Design review of the part built by this model. Coordinates are the model's own, in mm. Round coordinates to 2 decimals unless told otherwise and drop trailing zeros. Order: outer loops, then holes, each group sorted by start corner. A loop starts at its lowest first (then second) coordinate and runs counter-clockwise, first axis right, second up. Notation, with made-up numbers: M 47,-0.5 L 54,-0.5 A19 cw 54,17.5 Z; hole C -13,54.25 d7. An arc over 180 degrees is marked long. Write each question's results on one line, items separated by ' | '. Start each with the question number.
Item 1: Clearance check with a flat-ended pin moving along its axis: pin 1 (3.5 mm diameter, centred on x = -29.5, z = 36.51, fed in from -Y). State where the tip first meets the part, or that it passes through.
Item 2: Take a section at B-B, the plane z = 38.1. Write out the cut boundary in (x, y).
Item 3: Take a section at D-D, the plane y = 2.5. Count the separate pieces of the cut face and the enclosed holes in it, plus the area to 3 significant figures.
Item 4: Take a section at A-A, the plane x = 50.8. Write out the cut boundary in (y, z).
Item 5: Wall thickness on line 1 (Z direction, x = -34.5, y = 3.75); line 2 (Z direction, x = -29.5, y = 2.25); line 3 (X direction, y = 4.5, z = -3): over which ranges is each line inside the solid? List them lowest first. Write a range as [from, to].
Item 6: Take a section at C-C, the plane x = -29.5. Write out the cut boundary in (y, z).
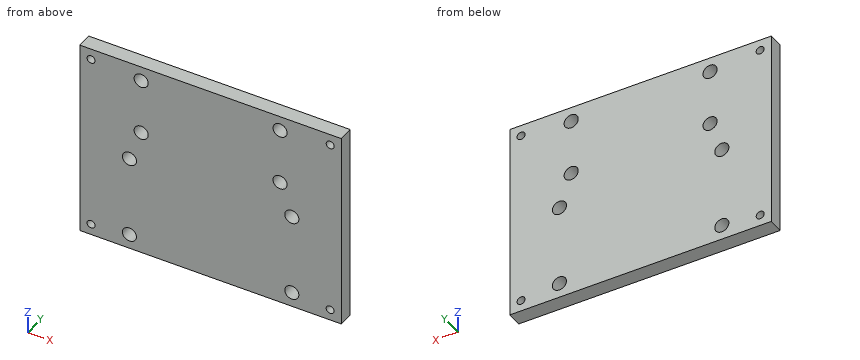
```python
from build123d import *

# Parameters (mm, degrees)
SKETCH1_W            = 111.125
SKETCH1_H            = 85.725
BOSS_EXTRUDE1_DEPTH  = 6.35
M3_CLEARANCE_HOLE1_D = 3.4
SKETCH3_R            = 3
CUT_EXTRUDE1_DEPTH   = 7.35


with BuildPart() as part:
    # Sketch1 → Boss-Extrude1 (new body)
    with BuildSketch(Plane(origin=(0, 0, 0), x_dir=(1, 0, 0), z_dir=(0, 1, 0))):
        Rectangle(SKETCH1_W, SKETCH1_H)
    extrude(amount=BOSS_EXTRUDE1_DEPTH)

    # M3 Clearance Hole1 (through all)
    with Locations(Plane(origin=(-50.8, 0, 38.1), x_dir=(0, 0, -1), z_dir=(0, -1, 0))):
        with Locations((0, 0), (0, 101.6), (76.2, 0), (76.2, 101.6)):
            Hole(M3_CLEARANCE_HOLE1_D / 2)

    # Sketch3 → Cut-Extrude1 (cut, through all)
    with BuildSketch(Plane(origin=(0, 6.35, 0), x_dir=(1, 0, 0), z_dir=(0, 1, 0))):
        with Locations((-34.5, 36.5125)):
            Circle(SKETCH3_R)
        with Locations((34.5, 36.5125)):
            Circle(SKETCH3_R)
        with Locations((34.5, 1.5125)):
            Circle(SKETCH3_R)
        with Locations((-34.5, 1.5125)):
            Circle(SKETCH3_R)
        with Locations((-29.5, -12.5125)):
            Circle(SKETCH3_R)
        with Locations((-29.5, -36.5125)):
            Circle(SKETCH3_R)
        with Locations((29.5, -36.5125)):
            Circle(SKETCH3_R)
        with Locations((29.5, -12.5125)):
            Circle(SKETCH3_R)
    extrude(amount=-CUT_EXTRUDE1_DEPTH, mode=Mode.SUBTRACT)


solid = part.part
```
Results list:
1) pin 1: through
2) outline: M -55.56,0 L -52.5,0 L -52.5,6.35 L -55.56,6.35 Z; M -49.1,0 L -32.05,0 L -32.05,6.35 L -49.1,6.35 Z; M -26.95,0 L 26.95,0 L 26.95,6.35 L -26.95,6.35 Z; M 32.05,0 L 49.1,0 L 49.1,6.35 L 32.05,6.35 Z; M 52.5,0 L 55.56,0 L 55.56,6.35 L 52.5,6.35 Z
3) separate pieces: 1 | enclosed holes: 12 | area: 9,260 mm²
4) outline: M 0,-42.86 L 6.35,-42.86 L 6.35,-39.8 L 0,-39.8 Z; M 0,-36.4 L 6.35,-36.4 L 6.35,36.4 L 0,36.4 Z; M 0,39.8 L 6.35,39.8 L 6.35,42.86 L 0,42.86 Z
5) line 1: [-42.86, -39.51], [-33.51, -4.51], [1.49, 42.86] | line 2: [-42.86, 9.51], [15.51, 33.51], [39.51, 42.86] | line 3: [-55.56, -37.11], [-31.89, 31.89], [37.11, 55.56]
6) outline: M 0,-42.86 L 6.35,-42.86 L 6.35,9.51 L 0,9.51 Z; M 0,15.51 L 6.35,15.51 L 6.35,33.51 L 0,33.51 Z; M 0,39.51 L 6.35,39.51 L 6.35,42.86 L 0,42.86 Z
